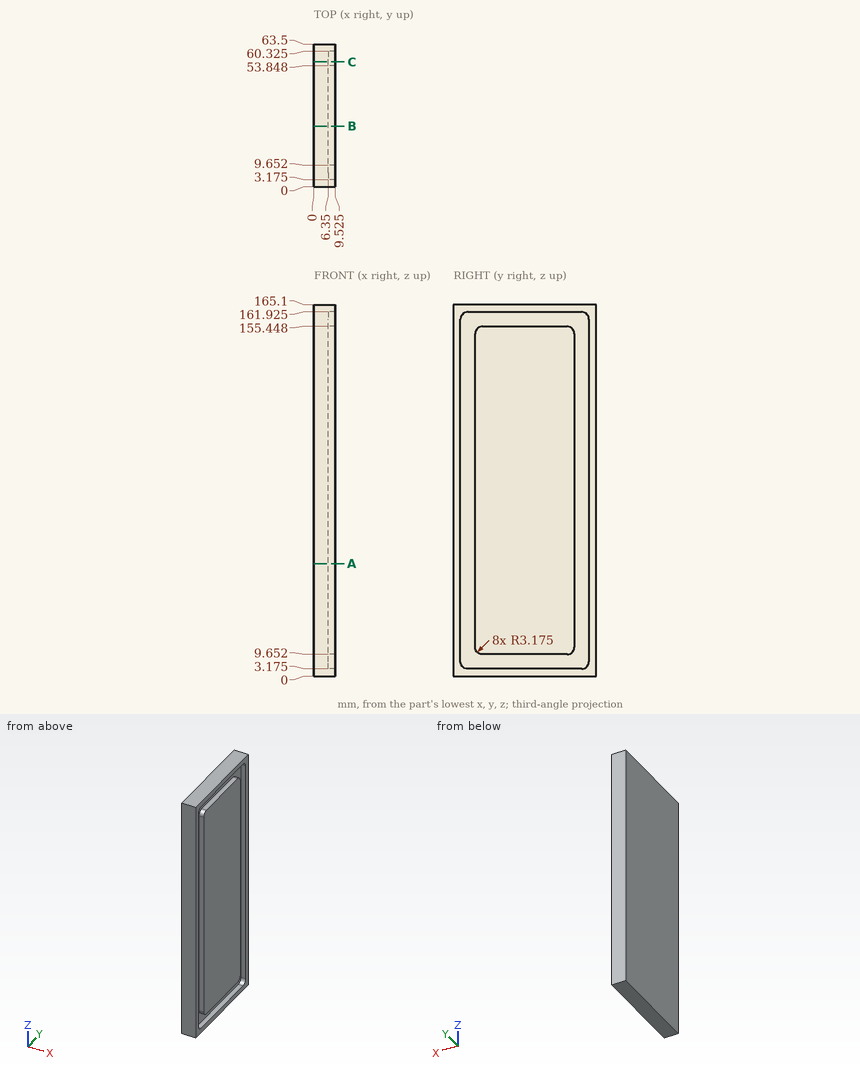
Input: dimensioned drawing with shaded views. Units: mm. Origin: part minimum x, y, z. Round coordinates to 2 decimals unless told otherwise and drop trailing zeros. Loops run counter-clockwise (first coordinate to the right, second up) from the corner with the lowest first, then second, coordinate; pieces in that order, holes last. Notation, with made-up numbers: (15, 34) -> (30, 34) arc R15 cw to (30, 60) -> close; hole circle Ø2 at (59.25, -1). An arc over 180 degrees is marked (long way). Use one line per item in the form item = value. Start each with the question number.
1) Section A-A on z = 50. Output: boundary loops of the cut face in (x, y) (3 decimals), then the cut area to 3 significant figures.
2) Section C-C on y = 55.5. Output: boundary loops of the cut face in (x, z) (3 decimals), then the cut area to 3 significant figures.
3) Section B-B on y = 27. Output: boundary loops of the cut face in (x, z) (3 decimals), then the cut area to 3 significant figures.
4) Line query: L1, parallel to Y at x = 7.25, z = 53 (3 decimals); L2, parallel to Z at x = 8.5, y = 17 (3 decimals). Output: solid intervals per line, ascending.
Response:
q1.outline = (0, 0) -> (9.525, 0) -> (9.525, 3.175) -> (6.35, 3.175) -> (6.35, 9.652) -> (9.525, 9.652) -> (9.525, 53.848) -> (6.35, 53.848) -> (6.35, 60.325) -> (9.525, 60.325) -> (9.525, 63.5) -> (0, 63.5) -> close
q1.area = 564 mm^2
q2.outline = (0, 0) -> (9.525, 0) -> (9.525, 3.175) -> (6.35, 3.175) -> (6.35, 161.925) -> (9.525, 161.925) -> (9.525, 165.1) -> (0, 165.1) -> close
q2.area = 1,070 mm^2
q3.outline = (0, 0) -> (9.525, 0) -> (9.525, 3.175) -> (6.35, 3.175) -> (6.35, 9.652) -> (9.525, 9.652) -> (9.525, 155.448) -> (6.35, 155.448) -> (6.35, 161.925) -> (9.525, 161.925) -> (9.525, 165.1) -> (0, 165.1) -> close
q3.area = 1,530 mm^2
q4.L1 = 0 to 3.175, 9.652 to 53.848, 60.325 to 63.5
q4.L2 = 0 to 3.175, 9.652 to 155.448, 161.925 to 165.1
